Read the model definition and answer for the solid it produces. Units are mm, in the model's axes. Face numbers are marked on the shaded views. A direction names the side the tool comes from. Give positions to 0.01 mm unless a question says otherwise; leave off trailing zeros. Order: outer loops, then holes, each group sorted by start corner. A loop starts at its lowest first (then second) coordinate and runs counter-clockwise, first axis right, second up.
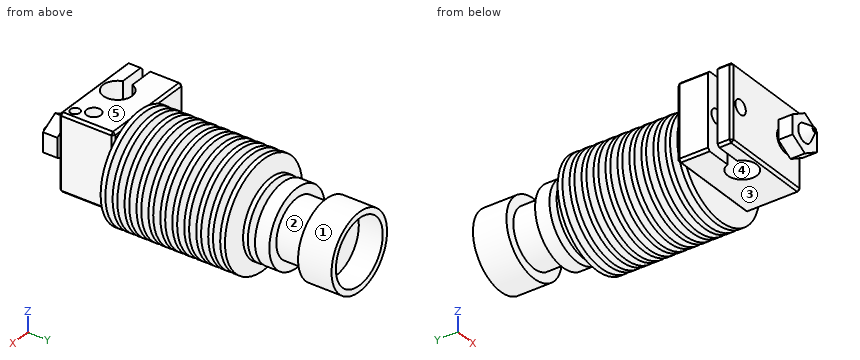
```python
from build123d import *

# Parameters (mm, degrees)
BOSS_EXTRUDE1_DEPTH              = 3
SKETCH2_R                        = 2.5
BOSS_EXTRUDE2_DEPTH              = 1
SKETCH3_W                        = 20
SKETCH3_H                        = 16
BOSS_EXTRUDE3_DEPTH              = 11.5
CUT_EXTRUDE1_DEPTH               = 17
SKETCH5_W                        = 3.025
SKETCH5_H                        = 16
SKETCH8_W                        = 1.5
SKETCH8_H                        = 54.6
F_3_0_3_DIAMETER_HOLE2_D         = 3
F_3_0_3_DIAMETER_HOLE2_DEPTH     = 3.45
F_3_0_3_DIAMETER_HOLE3_D         = 3
F_3_0_3_DIAMETER_HOLE3_DEPTH     = 59.6
M2X0_4_TAPPED_HOLE1_D            = 1.55
M2X0_4_TAPPED_HOLE1_DEPTH        = 4.45
M2X0_4_TAPPED_HOLE1_CBORE_D      = 2
M2X0_4_TAPPED_HOLE1_CBORE_DEPTH  = 2
F_0_4_0_4_DIAMETER_HOLE1_D       = 0.4
F_0_4_0_4_DIAMETER_HOLE1_DEPTH   = 3
F_13_5_13_5_DIAMETER_HOLE1_D     = 13.5
F_13_5_13_5_DIAMETER_HOLE1_DEPTH = 5
CHAMFER1_SIZE                    = 0.5


with BuildPart() as part:
    # Sketch1 → Boss-Extrude1 (new body)
    with BuildSketch(Plane.XZ.offset(42.25)):
        Polygon((-3.5, 2.020725942), (-3.5, -2.020725942), (0, -4.041451884), (3.5, -2.020725942), (3.5, 2.020725942), (0, 4.041451884), align=None)
    extrude(amount=-BOSS_EXTRUDE1_DEPTH)

    # Sketch2 → Boss-Extrude2 (add)
    with BuildSketch(Plane(origin=(0, -39.25, 0), x_dir=(-1, 0, 0), z_dir=(0, 1, 0))):
        Circle(SKETCH2_R)
    extrude(amount=BOSS_EXTRUDE2_DEPTH)

    # Sketch3 → Boss-Extrude3 (add)
    with BuildSketch(Plane.XZ.offset(38.25)):
        with Locations((-5.5, 0)):
            Rectangle(SKETCH3_W, SKETCH3_H)
    extrude(amount=-BOSS_EXTRUDE3_DEPTH)

    # Sketch4 → Cut-Extrude1 (cut, through all)
    with BuildSketch(Plane(origin=(0, 0, -8), x_dir=(-1, 0, 0), z_dir=(0, 0, -1))):
        with BuildLine():
            Line((15.5, -33.25), (9.854929947, -33.25))
            ThreePointArc((9.854929947, -33.25), (10.025, -34.25), (9.854929947, -35.25))
            Line((9.854929947, -35.25), (15.5, -35.25))
            Line((15.5, -35.25), (15.5, -33.25))
        make_face()
    extrude(amount=-CUT_EXTRUDE1_DEPTH, mode=Mode.SUBTRACT)

    # Sketch5 → Cut-Revolve1 (revolve, cut)
    with BuildSketch(Plane.XZ.offset(34.25)):
        with Locations((-5.4875, 0)):
            Rectangle(SKETCH5_W, SKETCH5_H)
    revolve(axis=Axis((-7, -34.25, 8), (0, 0, -1)), mode=Mode.SUBTRACT)

    # Sketch6 → Revolve1 (revolve)
    with BuildSketch(Plane.XY):
        Polygon((1.9, -42.249999999), (0, -42.249999999), (0, -44.25), (0.500000001, -44.25), align=None)
    revolve(axis=Axis((0, -42.249999999, 0), (0, -1, 0)))

    # Sketch7 → Revolve2 (revolve)
    with BuildSketch(Plane.XY):
        Polygon((8, 21.35), (0, 21.35), (0, -26.75), (2, -26.75), (2, -24.65), (11.15, -24.65), (11.15, -23.65), (7, -23.65), (7, -22.15), (11.15, -22.15), (11.15, -21.15), (6.75, -21.15), (6.75, -19.65), (11.15, -19.65), (11.15, -18.65), (6.5, -18.65), (6.5, -17.15), (11.15, -17.15), (11.15, -16.15), (6.25, -16.15), (6.25, -14.65), (11.15, -14.65), (11.15, -13.65), (6, -13.65), (6, -12.15), (11.15, -12.15), (11.15, -11.15), (5.75, -11.15), (5.75, -9.65), (11.15, -9.65), (11.15, -8.65), (5.5, -8.65), (5.5, -7.15), (11.15, -7.15), (11.15, -6.15), (5.25, -6.15), (5.25, -4.65), (11.15, -4.65), (11.15, -3.65), (5, -3.65), (5, -2.15), (11.15, -2.15), (11.15, -1.15), (4.75, -1.15), (4.75, 0.35), (11.15, 0.35), (11.15, 1.35), (4.5, 1.35), (4.5, 2.85), (8, 2.85), (8, 3.85), (4.5, 3.85), (4.5, 5.35), (8, 5.35), (8, 8.35), (6, 8.35), (6, 14.35), (8, 14.35), align=None)
    revolve(axis=Axis((0, 21.35, 0), (0, -1, 0)))

    # Sketch8 → Ø3.0 (3) Diameter Hole1 (revolve, cut)
    with BuildSketch(Plane(origin=(-13, -33.25, 0), x_dir=(0, 0, -1), z_dir=(1, 0, 0))):
        with Locations((0.75, 27.3)):
            Rectangle(SKETCH8_W, SKETCH8_H)
    revolve(axis=Axis((-13, -39.6, 0), (0, 1, 0)), mode=Mode.SUBTRACT)

    # Ø3.0 (3) Diameter Hole2
    with Locations(Plane.XY.offset(8)):
        with Locations((1, -33.45)):
            Hole(F_3_0_3_DIAMETER_HOLE2_D / 2, depth=F_3_0_3_DIAMETER_HOLE2_DEPTH)

    # Ø3.0 (3) Diameter Hole3
    with Locations(Plane(origin=(0, -38.25, 0), x_dir=(-1, 0, 0), z_dir=(0, -1, 0))):
        with Locations((13, 0)):
            Hole(F_3_0_3_DIAMETER_HOLE3_D / 2, depth=F_3_0_3_DIAMETER_HOLE3_DEPTH)

    # M2x0.4 Tapped Hole1
    with Locations(Plane.XY.offset(8)):
        with Locations((2.5, -36.25)):
            CounterBoreHole(M2X0_4_TAPPED_HOLE1_D / 2, M2X0_4_TAPPED_HOLE1_CBORE_D / 2, M2X0_4_TAPPED_HOLE1_CBORE_DEPTH, depth=M2X0_4_TAPPED_HOLE1_DEPTH)

    # Ø0.4 (0.4) Diameter Hole1
    with Locations(Plane(origin=(0, -44.25, 0), x_dir=(-1, 0, 0), z_dir=(0, -1, 0))):
        with Locations((0, 0)):
            Hole(F_0_4_0_4_DIAMETER_HOLE1_D / 2, depth=F_0_4_0_4_DIAMETER_HOLE1_DEPTH)

    # Ø13.5 (13.5) Diameter Hole1
    with Locations(Plane(origin=(0, 21.35, 0), x_dir=(1, 0, 0), z_dir=(0, 1, 0))):
        with Locations((0, 0)):
            Hole(F_13_5_13_5_DIAMETER_HOLE1_D / 2, depth=F_13_5_13_5_DIAMETER_HOLE1_DEPTH)

    # Chamfer1
    chamfer1_edges = [part.edges().sort_by_distance(p)[0] for p in [
        (-15.5, -26.75, 0),
        (-15.5, -30, -8),
        (-5.5, -26.75, 8),
        (-15.5, -30, 8),
        (4.5, -26.75, 0),
        (4.5, -32.5, 8),
        (-5.5, -26.75, -8),
        (4.5, -32.5, -8),
        (-15.5, -38.25, 0),
        (-5.5, -38.25, -8),
        (4.5, -38.25, 0),
        (-5.5, -38.25, 8),
        (-15.5, -36.75, -8),
        (-15.5, -36.75, 8),
    ]]
    chamfer(chamfer1_edges, length=CHAMFER1_SIZE)


solid = part.part
```
1) Given pin 1 (2.5 mm diameter, centred on x = 2.5, y = -36.25, fed in from +Z); pin 2 (0.6 mm diameter, centred on x = 3, y = -36.5, fed in from +Z); pin 3 (3 mm diameter, centred on y = -6, z = -3.5, fed in from -X), each flat-ended and moving along its own axis, determine where each tip first touches the part or whether it passes through.
Final values:
pin 1: stops at z = 8
pin 2: stops at z = 6
pin 3: stops at x = -10.97
2) For a pull along Y with two mould halves and no side action, classify the marked faces 4 and 5 as released by +Y, released by -Y, zero draft, split by the parting line, or undercut.
Final values:
face 4: undercut
face 5: zero draft
3) Consider L1, parallel to Y at x = -0.5, z = 2.75; L2, parallel to Z at x = -13, y = -28.5; L3, parallel to Y at x = -0.5, z = -2.25. Determine where each line is inside the solid, lowest interval first.
Final values:
L1: y = -42.25 to -39.25, -38.25 to -26.75, -24.65 to 16.35
L2: z = -8 to -1.5, 1.5 to 8
L3: y = -42.25 to -26.75, -24.65 to 16.35
4) The part is cut by section C-C on y = -34.25. Determine the outline of the cut face in (x, z) (3 decimals).
Final values:
outline: (-3.975, -8) - (4, -8) - (4.5, -7.5) - (4.5, 7.5) - (4, 8) - (2.269, 8) - (2.269, 4.55) - (-0.269, 4.55) - (-0.269, 8) - (-3.975, 8) - close
5) The part is cut by section A-A on y = 7.5. Determine the outline of the cut face in (x, z).
Final values:
outline: circle Ø16 at (0, 0)
6) The part is cut by section B-B on x = 8.75. Count the separate pieces of the cut face and the enclosed holes in it, and give its area (3 significant figures).
Final values:
separate pieces: 11
enclosed holes: 0
area: 152 mm2
7) A tool of negligible diameter and unlimited length cuts with its end or side. For the marked faces 1, 2 and 3, from which of +Z, -Z, +X, -X, +Y, -Y can it reach the whole face along a straight path? Write none if from no direction.
Final values:
face 1: +Y
face 2: none
face 3: -Z, +X, -X, -Y
